The model under review builds one solid part; all positions refer to its coordinate system, in mm. A direction names the side the tool comes from. Give positions to 0.01 mm unless a question says otherwise; leave off trailing zeros. Loops run counter-clockwise (first coordinate to the right, second up) from the corner with the lowest first, then second, coordinate; pieces in that order, holes last. Notation, with made-up numbers: (36.5, -11) - (81.5, -11) arc R20 ccw to (81.5, 17) - close; hole circle Ø11 at (-31, -24.5). An arc over 180 degrees is marked (long way). Return JSON: item names as keys, results as strings. Group by question number.
```python
from build123d import *

# Parameters (mm, degrees)
CROQUIS1_R              = 3.05
CROQUIS1_W              = 9.5
CROQUIS1_H              = 2.3
SALIENTE_EXTRUIR1_DEPTH = 3


with BuildPart() as part:
    # Croquis1 → Saliente-Extruir1 (new body)
    with BuildSketch(Plane(origin=(0, 0, 0), x_dir=(0, 0, -1), z_dir=(1, 0, 0))):
        Polygon((-14.9, -25), (-5.1, -25), (-5.1, -28.2), (5.1, -28.2), (5.1, -25), (14.9, -25), (14.9, -28.2), (25.1, -28.2), (25.1, -25), (40, -25), (40, 25), (-40, 25), (-40, -25), (-25.1, -25), (-25.1, -28.2), (-14.9, -28.2), align=None)
        with Locations((0, 6)):
            Circle(CROQUIS1_R, mode=Mode.SUBTRACT)
        with Locations((-20, 21.35)):
            Rectangle(CROQUIS1_W, CROQUIS1_H, mode=Mode.SUBTRACT)
        with Locations((0, 21.35)):
            Rectangle(CROQUIS1_W, CROQUIS1_H, mode=Mode.SUBTRACT)
        with Locations((20, 21.35)):
            Rectangle(CROQUIS1_W, CROQUIS1_H, mode=Mode.SUBTRACT)
    extrude(amount=SALIENTE_EXTRUIR1_DEPTH)


solid = part.part
```
1) We need section A-A, the plane z = 0. Write out the cut boundary in (x, y), plus the area to 3 significant figures.
2) We need section C-C, the plane x = 1. Count the separate pieces of the cut face and the enclosed holes in it, plus the area to 3 significant figures.
3) To check wall thickness, follow line 1 (Y direction, x = 1.4, z = 0); line 2 (Z direction, x = 2.85, y = 22); line 3 (Y direction, x = 2.55, z = 16). State the ranges of each line that lie inside material, in increasing order.
4) Draft analysis for pull direction Y (two halves, no side actions). For faces 4 (the face through (1, 20.2, 20)), 5 (the face through (1, -27, 25.1)), 6 (the face through (1, 25, -1)), 7 (the face through (1, -28.2, 20)), state which applies: +Y half, -Y half, draft (parallel to the pull), parting line (faces both ways), or undercut.
5) For pin 1 Ø1.5 at (x, y) = (1, -26) entering from -Z, flat-tipped, find the tip position at first contact; note if it passes through.
6) Tool access review of faces 1 (the face through (1, -27, -14.9)), 2 (the face through (1, -27, -25.1)), 3 (the face through (1, 22.5, 0)): name each direction out of +Z, -Z, +X, -X, +Y, -Y from which nothing blocks a thin tool from reaching the whole face with its end or side.
7) We need section B-B, the plane y = 6. Write out the cut boundary in (x, z).
Findings:
{
 "1": {"outline": "(0, -28.2) - (3, -28.2) - (3, 2.95) - (0, 2.95) - close; (0, 9.05) - (3, 9.05) - (3, 20.2) - (0, 20.2) - close; (0, 22.5) - (3, 22.5) - (3, 25) - (0, 25) - close", "area": "134 mm^2"},
 "2": {"separate pieces": "1", "enclosed holes": "4", "area": "4,000 mm^2"},
 "3": {"line 1": "y = -28.2 to 2.95, 9.05 to 20.2, 22.5 to 25", "line 2": "z = -40 to -24.75, -15.25 to -4.75, 4.75 to 15.25, 24.75 to 40", "line 3": "y = -28.2 to 20.2, 22.5 to 25"},
 "4": {"face 4": "undercut", "face 5": "draft", "face 6": "+Y half", "face 7": "-Y half"},
 "5": {"pin 1": "stops at z = -25.1"},
 "6": {"face 1": "+X, -X, -Y", "face 2": "-Z, +X, -X, -Y", "face 3": "+X, -X"},
 "7": {"outline": "(0, -40) - (3, -40) - (3, -3.05) - (0, -3.05) - close; (0, 3.05) - (3, 3.05) - (3, 40) - (0, 40) - close"}
}
